Could you check a few things on this model? Use its own coordinates, in mm. A direction names the side the tool comes from. Round coordinates to 2 decimals unless told otherwise and drop trailing zeros. Write each loop counter-clockwise with the first axis right and the second up, starting at its lowest first coordinate (ties: lowest second). Pieces come first, ordered by that corner, then holes. Notation, with made-up numbers: (-7, 1.25) -> (22, 1.25) arc R16 cw to (22, 7.25) -> close; hole circle Ø3 at (32.5, 62.5). An arc over 180 degrees is marked (long way). Answer as CSV lines item,"result". Start each with the question number.
Q1. Will these pins go through, and if not, where does the flat tip stop? pin 1 Ø15.5 at (x, y) = (-89, -53.5) entering from +Z; pin 2 Ø10 at (x, y) = (-48.5, -110) entering from +Z; pin 3 Ø23 at (y, z) = (-47, 37) entering from +X; pin 4 Ø1.5 at (y, z) = (-69, 51) entering from -X.
Q2. If we mould it in two halves opening along Y, with no side actions, what happens to faces 6 (the flat face through (-11, -48, 0)), 7 (the flat face through (7, -83.778, -25)), 8 (the flat face through (-59, -127, -1)), 9 (the flat face through (-101, -22.009, 64))? For each: pulls with the +Y half, pulls with the -Y half, needs draft (parallel to the pull), parting line crosses it, or undercut.
Q3. Imagine slicing it at D-D on x = -102. Please give me the cut outline in (y, z).
Q4. Imagine slicing it at C-C on y = -56. Please give me the cut outline in (x, z).
Q5. If I drill on line 1 (Y direction, x = 23, z = -3); line 2 (Y direction, x = -90.5, z = 52); line 3 (X direction, y = -65.5, z = -9.5), over which ranges is the centre line in solid material (lowest first)? Write a range as [from, to].
Q6. For faces 1 (the flat face through (-75, -63, 29)), 2 (the flat face through (-35.832, -67, -25)), 3 (the flat face through (-39, -63, -50.8)), 4 (the flat face through (-101, -112, 76.2)), 5 (the flat face through (-101, -59, 50.8)), which set-ups out of +Z, -Z, +X, -X, +Y, -Y let a thin tool reach every point of the face, with its end or its side?
Q7. Imagine slicing it at A-A on z = 54.5. Please give me the cut outline in (x, y), and give its area (3 significant figures).
Q8. Imagine slicing it at B-B on x = 22.5. Please give me the cut outline in (y, z), and give its area (3 significant figures).
from build123d import *

# Parameters (mm, degrees)
F1_DEPTH = 127
F2_W     = 51.9999986213
F2_H     = 75.4991620779
F3_DEPTH = 25.4
F4_W     = 87.8321913701
F4_H     = 34.6736311913
F5_DEPTH = 77.47


with BuildPart() as f1:
    # F0 (on Front) → F1 (new body)
    with BuildSketch(Plane.XZ):
        Polygon((-75.0000013787, 76.2), (-127, 76.2), (-127, -50.8), (51.9999986213, -50.8), (51.9999986213, 0), (-75.0000013787, 0), align=None)
    extrude(amount=F1_DEPTH)

    # F2 (on face) → F3 (cut)
    with BuildSketch(Plane.XY.offset(76.2)):
        with Locations((-101.0000006893, -59.7584694624)):
            Rectangle(F2_W, F2_H)
    extrude(amount=-F3_DEPTH, mode=Mode.SUBTRACT)

    # F4 (on face) → F5 (cut)
    with BuildSketch(Plane.XY):
        with Locations((8.0839029363, -66.4408057928)):
            Rectangle(F4_W, F4_H)
    extrude(amount=-F5_DEPTH, mode=Mode.SUBTRACT)


solid = f1.part
Checks:
1,pin 1,"z = 50.8"
1,pin 2,"z = 0"
1,pin 3,"x = -75"
1,pin 4,"x = -127"
2,face 6,"needs draft"
2,face 7,"undercut"
2,face 8,"pulls with the -Y half"
2,face 9,"undercut"
3,outline,"(-127, -50.8) -> (0, -50.8) -> (0, 76.2) -> (-22.01, 76.2) -> (-22.01, 50.8) -> (-97.51, 50.8) -> (-97.51, 76.2) -> (-127, 76.2) -> close"
4,outline,"(-127, -50.8) -> (-35.83, -50.8) -> (-35.83, 0) -> (-75, 0) -> (-75, 50.8) -> (-127, 50.8) -> close"
5,line 1,"[-127, -83.78], [-49.1, 0]"
5,line 2,"[-127, -97.51], [-22.01, 0]"
5,line 3,"[-127, -35.83]"
6,face 1,"+Z, +X, +Y, -Y"
6,face 2,"+Z, -Z, +X"
6,face 3,"-Z, +X, -X, +Y, -Y"
6,face 4,"+Z, +X, -X, +Y, -Y"
6,face 5,"+Z, +X, -X"
7,outline,"(-127, -127) -> (-75, -127) -> (-75, -97.51) -> (-127, -97.51) -> close; (-127, -22.01) -> (-75, -22.01) -> (-75, 0) -> (-127, 0) -> close"
7,area,"2,680 mm^2"
8,outline,"(-127, -50.8) -> (-83.78, -50.8) -> (-83.78, 0) -> (-127, 0) -> close; (-49.1, -50.8) -> (0, -50.8) -> (0, 0) -> (-49.1, 0) -> close"
8,area,"4,690 mm^2"
